Geometry check sheet. Reference: drawing and pictorial views, mm from the part's lowest x, y, z. A direction names the side the tool comes from. Give positions to 0.01 mm unless a question says otherwise; leave off trailing zeros. Order: outer loops, then holes, each group sorted by start corner. A loop starts at its lowest first (then second) coordinate and runs counter-clockwise, first axis right, second up. Notation, with made-up numbers: M -11.75,14 L 3.25,14 A20 ccw 3.25,52 Z; hole C 59,49.5 d2. An arc over 180 degrees is marked long. Answer as a JSON object with one key per item and string values. Group by question number.
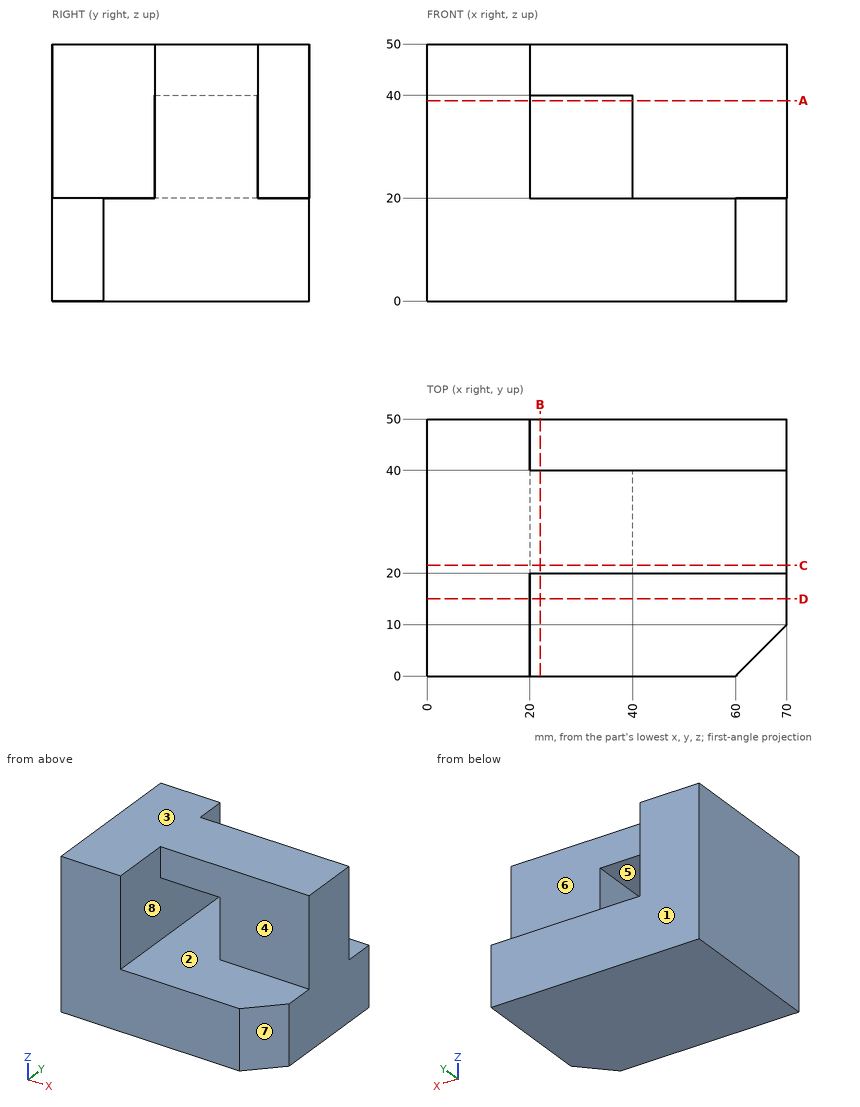
1. Cross-section at A-A (z = 39). Record the cut outline in (x, y).
2. Depth check by flat-ended pin: pin 1 (2 mm diameter, centred on x = 46.5, z = 35.5, fed in from -Y); pin 2 (1.5 mm diameter, centred on y = 13.5, z = 27, fed in from -X). Enter the tip coordinate at first touch or a pass-through.
3. Access from +Z, -Z, +X, -X, +Y, -Y to the whole of each face (thin tool, end or side, straight path). Record for the marked faces 1, 2, 3, 4 and 5.
4. Cross-section at C-C (y = 21.5). Record the cut outline in (x, z), and give its area (3 significant figures).
5. Cross-section at B-B (x = 22). Record the cut outline in (y, z).
6. Thickness scan on line 1 along Z through (x, y) = (25, 35); line 2 along X through (y, z) = (24, 39); line 3 along X through (y, z) = (5, 24). Record the ranges inside material, lowest first. Write a range as [from, to].
7. Release check for a two-part mould opening along X. For the marked faces 6, 7 and 8 record: released by +X, released by -X, zero draft, split by the parting line, or undercut.
8. Cross-section at D-D (y = 15). Record the cut outline in (x, z).
Report:
{
 "1": {"outline": "M 0,0 L 20,0 L 20,50 L 0,50 Z; M 40,20 L 70,20 L 70,40 L 40,40 Z"},
 "2": {"pin 1": "stops at y = 20", "pin 2": "stops at x = 0"},
 "3": {"face 1": "+Z, -Z, +X, -X, +Y", "face 2": "none", "face 3": "+Z, +X, -X, +Y, -Y", "face 4": "+Z, +X, -Y", "face 5": "+Y, -Y"},
 "4": {"outline": "M 0,0 L 70,0 L 70,50 L 0,50 Z; hole M 20,20 L 40,20 L 40,40 L 20,40 Z", "area": "3,100 mm2"},
 "5": {"outline": "M 0,0 L 50,0 L 50,20 L 0,20 Z; M 20,40 L 40,40 L 40,50 L 20,50 Z"},
 "6": {"line 1": "z = [0, 20], [40, 50]", "line 2": "x = [0, 20], [40, 70]", "line 3": "x = [0, 20]"},
 "7": {"face 6": "zero draft", "face 7": "released by +X", "face 8": "undercut"},
 "8": {"outline": "M 0,0 L 70,0 L 70,20 L 20,20 L 20,50 L 0,50 Z"}
}
